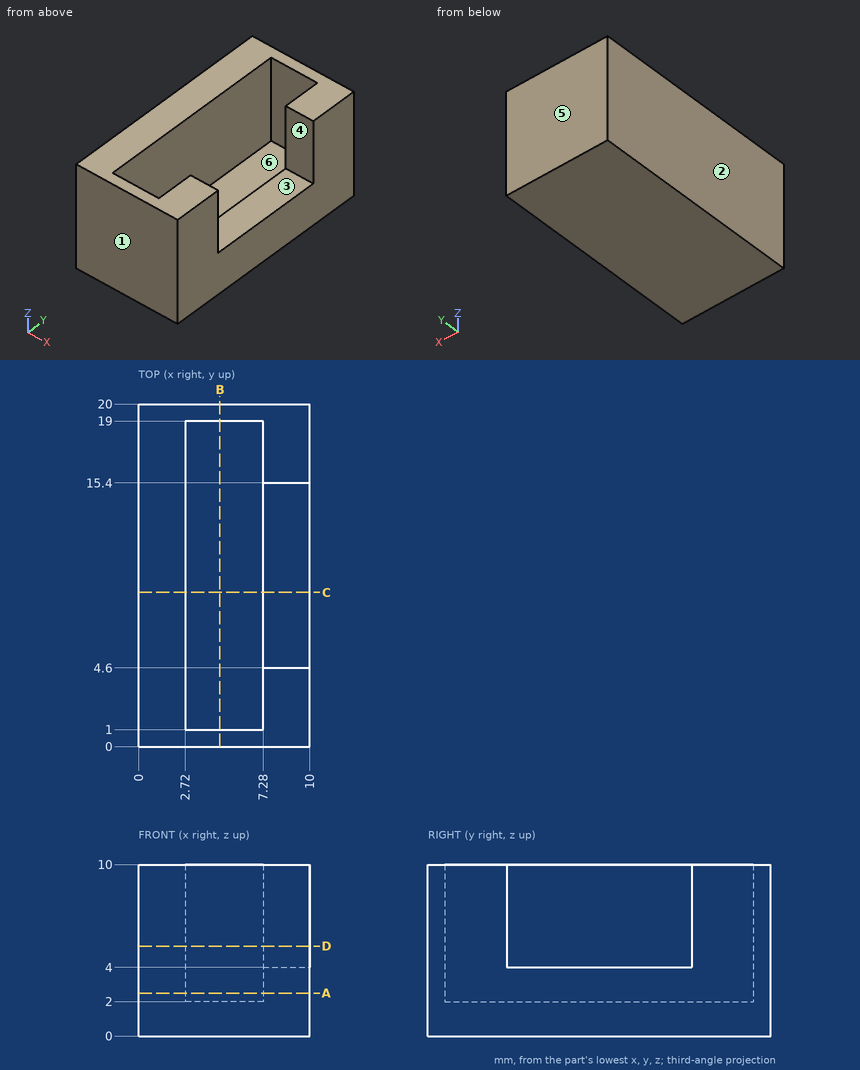
Print and shaded views of the part. All mm, measured from the part's lowest x, y and z. A direction names the side the tool comes from. Coordinates: 2 decimals unless noted, no trailing zeros. Order: outer loops, then holes, each group sorted by start corner. A loop starts at its lowest first (then second) coordinate and runs counter-clockwise, first axis right, second up. Notation, with made-up numbers: (-15.5, 87) -> (4.5, 87) arc R17 ccw to (4.5, 104) -> close; hole circle Ø8 at (50, 34). An arc over 180 degrees is marked (long way). Use one line per item in the form item = value. Start each with the question number.
1) Band-saw the part on D-D on z = 5.25. Give the cut face in (x, y).
2) Pull direction Y, two halves, no side cores. Call the marked faces 1, 2 and 3: +Y half, -Y half, draft (parallel to the pull), parting line (faces both ways), or undercut.
3) Band-saw the part on A-A on z = 2.5. Give the cut face in (x, y), then the cut area to 3 significant figures.
4) Drop flat-ended pins along their axis: pin 1 (2.5 mm diameter, centred on x = 5, z = 5, fed in from -Y); pin 2 (2 mm diameter, centred on x = 9, y = 12.5, fed in from +Z). Give the stop position or say it passes through.
5) Band-saw the part on B-B on x = 4.75. Give the cut face in (y, z).
6) Tool access for the marked faces 4, 5 and 6: list every direction of +Z, -Z, +X, -X, +Y, -Y with a clear straight run to the whole face (end or side of a thin tool).
7) Band-saw the part on C-C on y = 9. Give the cut face in (x, z), then the cut area to 3 significant figures.
8) Drill centre lines: L1, parallel to X at y = 10.25, z = 3.25; L2, parallel to Y at x = 5.25, z = 9.75; L3, parallel to Y at x = 9.25, z = 4.5. Where is each one in solid material? Low to high. Write a range as [from, to].
Entries:
q1.outline = (0, 0) -> (10, 0) -> (10, 4.6) -> (7.28, 4.6) -> (7.28, 1) -> (2.72, 1) -> (2.72, 19) -> (7.28, 19) -> (7.28, 15.4) -> (10, 15.4) -> (10, 20) -> (0, 20) -> close
q2.face_1 = -Y half
q2.face_2 = draft
q2.face_3 = undercut
q3.outline = (0, 0) -> (10, 0) -> (10, 20) -> (0, 20) -> close; hole (2.72, 1) -> (7.28, 1) -> (7.28, 19) -> (2.72, 19) -> close
q3.area = 118 mm2
q4.pin_1 = 0
q4.pin_2 = 4
q5.outline = (0, 0) -> (20, 0) -> (20, 10) -> (19, 10) -> (19, 2) -> (1, 2) -> (1, 10) -> (0, 10) -> close
q6.face_4 = +Z, +X
q6.face_5 = +Z, -Z, +X, -X, +Y
q6.face_6 = +Z
q7.outline = (0, 0) -> (10, 0) -> (10, 4) -> (7.28, 4) -> (7.28, 2) -> (2.72, 2) -> (2.72, 10) -> (0, 10) -> close
q7.area = 47.2 mm2
q8.L1 = [0, 2.72], [7.28, 10]
q8.L2 = [0, 1], [19, 20]
q8.L3 = [0, 4.6], [15.4, 20]
